Work out the finished part from the listing and answer in its coordinate system (mm). Give positions to 0.01 mm unless a question says otherwise; leave off trailing zeros. Loops run counter-clockwise (first coordinate to the right, second up) from the corner with the lowest first, then second, coordinate; pieces in that order, holes last.
```python
from build123d import *

# Parameters (mm, degrees)
F1_DEPTH = 5.08
F3_DEPTH = 3.175
F5_D     = 3.4544
F7_D     = 3.429
F8_R     = 36.195
F9_DEPTH = 5.081


with BuildPart() as f1:
    # F0 (on Top) → F1 (new body)
    with BuildSketch(Plane.XY):
        with BuildLine():
            ThreePointArc((0, 12.7), (3.7197438789, 3.7197438789), (12.7, 0))
            Line((12.7, 0), (152.4, 0))
            ThreePointArc((152.4, 0), (161.3802561211, 3.7197438789), (165.1, 12.7))
            Line((165.1, 12.7), (165.1, 177.8))
            ThreePointArc((165.1, 177.8), (161.3802561211, 186.7802561211), (152.4, 190.5))
            Line((152.4, 190.5), (12.7, 190.5))
            ThreePointArc((12.7, 190.5), (3.7197438789, 186.7802561211), (0, 177.8))
            Line((0, 177.8), (0, 12.7))
        make_face()
        with BuildLine():
            ThreePointArc((12.7, 158.75), (18.2796158184, 172.2203841816), (31.75, 177.8))
            Line((31.75, 177.8), (133.35, 177.8))
            ThreePointArc((133.35, 177.8), (146.8203841816, 172.2203841816), (152.4, 158.75))
            Line((152.4, 158.75), (152.4, 31.75))
            ThreePointArc((152.4, 31.75), (146.8203841816, 18.2796158184), (133.35, 12.7))
            Line((133.35, 12.7), (31.75, 12.7))
            ThreePointArc((31.75, 12.7), (18.2796158184, 18.2796158184), (12.7, 31.75))
            Line((12.7, 31.75), (12.7, 158.75))
        make_face(mode=Mode.SUBTRACT)
    extrude(amount=F1_DEPTH)

    # F2 (on face) → F3 (cut)
    with BuildSketch(Plane.XY.offset(5.08)):
        with BuildLine():
            ThreePointArc((3.175, 30.1498), (11.0757359988, 11.0757359988), (30.1498, 3.175))
            Line((30.1498, 3.175), (134.9502, 3.175))
            ThreePointArc((134.9502, 3.175), (154.0242640012, 11.0757359988), (161.925, 30.1498))
            Line((161.925, 30.1498), (161.925, 160.3502))
            ThreePointArc((161.925, 160.3502), (154.0242640012, 179.4242640012), (134.9502, 187.325))
            Line((134.9502, 187.325), (30.1498, 187.325))
            ThreePointArc((30.1498, 187.325), (11.0757359988, 179.4242640012), (3.175, 160.3502))
            Line((3.175, 160.3502), (3.175, 30.1498))
        make_face()
        with BuildLine():
            ThreePointArc((30.1498, 8.763), (15.0270486921, 15.0270486921), (8.763, 30.1498))
            Line((8.763, 30.1498), (8.763, 160.3502))
            ThreePointArc((8.763, 160.3502), (15.0270486921, 175.4729513079), (30.1498, 181.737))
            Line((30.1498, 181.737), (134.9502, 181.737))
            ThreePointArc((134.9502, 181.737), (150.0729513079, 175.4729513079), (156.337, 160.3502))
            Line((156.337, 160.3502), (156.337, 30.1498))
            ThreePointArc((156.337, 30.1498), (150.0729513079, 15.0270486921), (134.9502, 8.763))
            Line((134.9502, 8.763), (30.1498, 8.763))
        make_face(mode=Mode.SUBTRACT)
    extrude(amount=-F3_DEPTH, mode=Mode.SUBTRACT)

    # F5 (through all)
    with Locations(Plane(origin=(0, 0, 0), x_dir=(1, 0, 0), z_dir=(0, 0, -1))):
        with Locations((8.2098719395, -182.2901280605), (156.8901280605, -182.2901280605), (156.8901280605, -8.2098719395), (8.2098719395, -8.2098719395)):
            Hole(F5_D / 2)

    # F7 (through all)
    with Locations(Plane.XY.offset(5.08)):
        with Locations((14.3002, 185.7248), (150.7998, 185.7248), (14.3002, 4.7752), (150.7998, 4.7752)):
            Hole(F7_D / 2)

    # F8 (on face) → F9 (cut, through all)
    with BuildSketch(Plane.XY.offset(5.08)):
        with Locations((79.0035873652, 142.875)):
            Circle(F8_R)
    extrude(amount=-F9_DEPTH, mode=Mode.SUBTRACT)


solid = f1.part
```
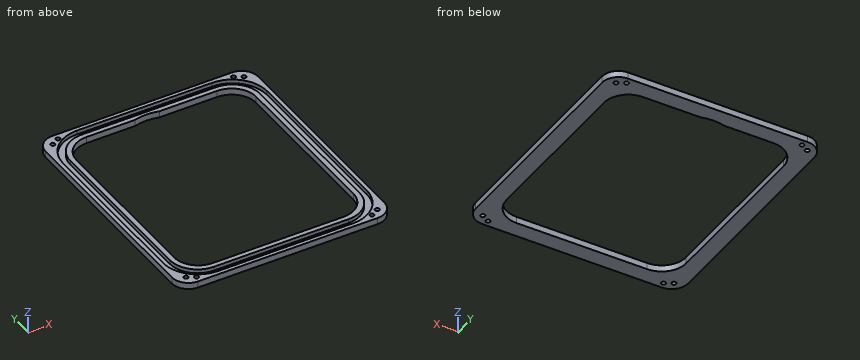
Q1. Section B-B on y = 83 is taken. Give the vertices of the cut face in (x, z) (3 decimals).
Q2. Section C-C on z = 0.9 is taken. State how many separate pieces and enclosed holes the cut face has, plus the area to 3 significant figures.
Q3. Consider line 1 along Y through (x, z) = (53.5, 2.3) (3 decimals); line 2 along X through (y, z) = (39, 4.1) (3 decimals); line 3 along Y through (x, z) = (70, 2.4) (3 decimals). Determine where each line is inside the solid, lowest interval first.
Q4. Section A-A on x = 113 is taken. Give the vertices of the cut face in (y, z) (3 decimals), plus the area to 3 significant figures.
Check result:
1. outline: (0, 0) - (12.7, 0) - (12.7, 5.08) - (8.763, 5.08) - (8.763, 1.905) - (3.175, 1.905) - (3.175, 5.08) - (0, 5.08) - close; (152.4, 0) - (165.1, 0) - (165.1, 5.08) - (161.925, 5.08) - (161.925, 1.905) - (156.337, 1.905) - (156.337, 5.08) - (152.4, 5.08) - close
2. separate pieces: 1
2. enclosed holes: 9
2. area: 8,470 mm2
3. line 1: y = 0 to 3.175, 8.763 to 12.7, 177.8 to 181.737, 187.325 to 190.5
3. line 2: x = 0 to 3.175, 8.763 to 12.7, 152.4 to 156.337, 161.925 to 165.1
3. line 3: y = 0 to 3.175, 8.763 to 12.7, 177.932 to 181.737, 187.325 to 190.5
4. outline: (0, 0) - (12.7, 0) - (12.7, 5.08) - (8.763, 5.08) - (8.763, 1.905) - (3.175, 1.905) - (3.175, 5.08) - (0, 5.08) - close; (177.8, 0) - (190.5, 0) - (190.5, 5.08) - (187.325, 5.08) - (187.325, 1.905) - (181.737, 1.905) - (181.737, 5.08) - (177.8, 5.08) - close
4. area: 93.5 mm2
